```python
from build123d import *

# Parameters (mm, degrees)
SKETCH1_R           = 1.875
SKETCH1_R_2         = 0.889
BOSS_EXTRUDE1_DEPTH = 8
SKETCH2_R           = 4
CUT_EXTRUDE1_DEPTH  = 5.5


with BuildPart() as part:
    # Sketch1 → Boss-Extrude1 (new body)
    with BuildSketch(Plane(origin=(0, 0, 0), x_dir=(1, 0, 0), z_dir=(0, 1, 0))):
        with BuildLine():
            Line((-7.071067812, 2.5), (-17.571067812, 2.5))
            Line((-17.571067812, 2.5), (-17.571067812, -2.5))
            Line((-17.571067812, -2.5), (-7.071067812, -2.5))
            ThreePointArc((-7.071067812, -2.5), (0, -7.5), (7.071067812, -2.5))
            Line((7.071067812, -2.5), (17.571067812, -2.5))
            Line((17.571067812, -2.5), (17.571067812, 2.5))
            Line((17.571067812, 2.5), (7.071067812, 2.5))
            ThreePointArc((7.071067812, 2.5), (0, 7.5), (-7.071067812, 2.5))
        make_face()
        with Locations(Location((0, 0, 0), (0, 0, 270))):
            Circle(SKETCH1_R, mode=Mode.SUBTRACT)
        with Locations(Location((-14.5, 0, 0), (0, 0, 270))):
            Circle(SKETCH1_R_2, mode=Mode.SUBTRACT)
        with Locations(Location((14.5, 0, 0), (0, 0, 270))):
            Circle(SKETCH1_R_2, mode=Mode.SUBTRACT)
    extrude(amount=BOSS_EXTRUDE1_DEPTH)

    # Sketch2 → Cut-Extrude1 (cut)
    with BuildSketch(Plane(origin=(0, 8, 0), x_dir=(1, 0, 0), z_dir=(0, 1, 0))):
        with Locations(Location((0, 0, 0), (0, 0, 270))):
            Circle(SKETCH2_R)
    extrude(amount=-CUT_EXTRUDE1_DEPTH, mode=Mode.SUBTRACT)


solid = part.part
```
Build history of the part. All positions in model axes, mm. A direction names the side the tool comes from. Round coordinates to 2 decimals unless told otherwise and drop trailing zeros. Order: outer loops, then holes, each group sorted by start corner. A loop starts at its lowest first (then second) coordinate and runs counter-clockwise, first axis right, second up. Notation, with made-up numbers: (59.25, 63) -> (65.25, 63) arc R16 ccw to (65.25, 87) -> close; hole circle Ø6 at (10.25, -5.75). An arc over 180 degrees is marked (long way). Answer in a Markdown table with one row per item.
1) Band-saw the part on D-D on y = 2. Give the cut face in (x, z) (3 decimals).
Values:
| item | result |
|---|---|
| outline | (-17.571, -2.5) -> (-7.071, -2.5) arc R7.5 ccw to (7.071, -2.5) -> (17.571, -2.5) -> (17.571, 2.5) -> (7.071, 2.5) arc R7.5 ccw to (-7.071, 2.5) -> (-17.571, 2.5) -> close; hole circle Ø1.778 at (-14.5, 0); hole circle Ø3.75 at (0, 0); hole circle Ø1.778 at (14.5, 0) |
2) Band-saw the part on A-A on x = 0. Give the cut face in (y, z) (3 decimals).
Values:
| item | result |
|---|---|
| outline | (0, -7.5) -> (8, -7.5) -> (8, -4) -> (2.5, -4) -> (2.5, -1.875) -> (0, -1.875) -> close; (0, 1.875) -> (2.5, 1.875) -> (2.5, 4) -> (8, 4) -> (8, 7.5) -> (0, 7.5) -> close |
3) Wall check: L1, parallel to X at y = 1.55, z = 0 (3 decimals); L2, parallel to X at y = 5.1, z = 0; L3, parallel to Z at x = 0, y = 1.5 (3 decimals). Give the ranges that are in metal, low to high.
Values:
| item | result |
|---|---|
| L1 | -17.571 to -15.389, -13.611 to -1.875, 1.875 to 13.611, 15.389 to 17.571 |
| L2 | -17.57 to -15.39, -13.61 to -4, 4 to 13.61, 15.39 to 17.57 |
| L3 | -7.5 to -1.875, 1.875 to 7.5 |
4) Pin check, flat tips, straight feed: P1, Ø4, axis at x = 12, y = 2.5, coming from the +Z side; P2, Ø4, axis at x = -0.5, z = -1.5, coming from the +Y side; P3, Ø4, axis at x = -14.5, y = 2, coming from the -Z side. Stop position of each tip, or through.
Values:
| item | result |
|---|---|
| P1 | z = 2.5 |
| P2 | y = 2.5 |
| P3 | z = -2.5 |
5) Band-saw the part on B-B on y = 3.75. Give the cut face in (x, z).
Values:
| item | result |
|---|---|
| outline | (-17.57, -2.5) -> (-7.07, -2.5) arc R7.5 ccw to (7.07, -2.5) -> (17.57, -2.5) -> (17.57, 2.5) -> (7.07, 2.5) arc R7.5 ccw to (-7.07, 2.5) -> (-17.57, 2.5) -> close; hole circle Ø1.78 at (-14.5, 0); hole circle Ø8 at (0, 0); hole circle Ø1.78 at (14.5, 0) |
6) Band-saw the part on C-C on x = 14.5. Give the cut face in (y, z), and give its area (3 significant figures).
Values:
| item | result |
|---|---|
| outline | (0, -2.5) -> (8, -2.5) -> (8, -0.89) -> (0, -0.89) -> close; (0, 0.89) -> (8, 0.89) -> (8, 2.5) -> (0, 2.5) -> close |
| area | 25.8 mm2 |
7) Which spindle directions (+Z, -Z, +X, -X, +Y, -Y) get a long thin tool onto all of the face, cutting with end or side? Do faces 1 (the flat face through (-12, 4, 2.5)), 2 (the flat face through (12, 4, -2.5)), 3 (the cylindrical face through (-3.905, 5.288, -0.867)), 4 (the flat face through (12, 4, 2.5)). Say none if no direction does.
Values:
| item | result |
|---|---|
| face 1 | +Z, -X, +Y, -Y |
| face 2 | -Z, +X, +Y, -Y |
| face 3 | +Y |
| face 4 | +Z, +X, +Y, -Y |
